The drawing under review shows one solid part. Ordinate dimensions are in mm from its lowest x, y, z. Give positions to 0.01 mm unless a question says otherwise; leave off trailing zeros. Loops run counter-clockwise (first coordinate to the right, second up) from the corner with the lowest first, then second, coordinate; pieces in that order, holes last.
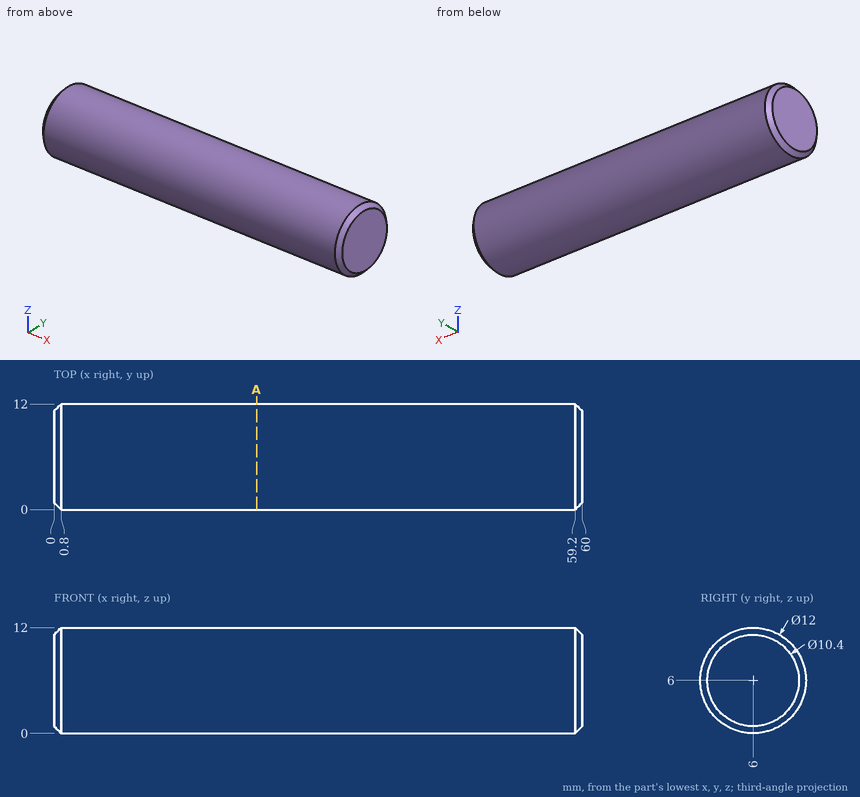
Item 1: Take a section at A-A on x = 23. Give the boundary of the cut face in (y, z), and give its area (3 significant figures).
Answer:
outline: circle Ø12 at (6, 6)
area: 113 mm2
Item 2: Clearance check with flat-ended pins moving along their axes: pin 1 Ø5 at (x, y) = (40, 8.5) entering from +Z; pin 2 Ø1 at (x, y) = (40, 9.5) entering from +Z; pin 3 Ø1.5 at (x, y) = (26, 3.5) entering from +Z; pin 4 Ø1 at (x, z) = (17.5, 8) entering from +Y. State where each tip first meets the part, or that it passes through.
Answer:
pin 1: stops at z = 12
pin 2: stops at z = 11.2
pin 3: stops at z = 11.74
pin 4: stops at y = 11.81
Item 3: For L1, parallel to Z at x = 57, y = 3; L2, parallel to Y at x = 25, z = 9.75, list the stretches that pass through material, from the lowest coordinate up.
Answer:
L1: z = 0.8 to 11.2
L2: y = 1.32 to 10.68
